Autodesk Fusion 360 part; units mm, degrees
sketch "Sketch1" plane through (0, 0, 0) normal (0, 0, 1) x (1, 0, 0)
  line L0 (0, 0) -> (169.51, 0)
  line L1 (169.51, 0) -> (169.51, 124.6)
  line L2 (169.51, 124.6) -> (0, 124.6)
  line L3 (0, 124.6) -> (0, 0)
  dimension "d1" = 169.51
  dimension "d2" = 124.6
extrude "Extrude1" add sketch "Sketch1" along normal blind 9.2 makes body 1
sketch "Sketch2" plane through (0, 0, 9.2) normal (0, 0, 1) x (-1, 0, 0)
  line L0 (0, -124.6) -> (0, 0)
  line L1 (0, 0) -> (-169.51, 0)
  line L2 (-169.51, 0) -> (-169.51, -124.6)
  line L3 (-169.51, -124.6) -> (0, -124.6)
  line L4 (-1.5, -10.3) -> (-168.01, -10.3)
  line L5 (-168.01, -10.3) -> (-168.01, -113)
  line L6 (-168.01, -113) -> (-1.5, -113)
  line L7 (-1.5, -113) -> (-1.5, -10.3)
  dimension "d5" = 1.5
  dimension "d6" = 1.5
  dimension "d7" = 11.6
  dimension "d8" = 10.3
extrude "Extrude2" cut sketch "Sketch2" against normal blind 7.6 contours L4 L5 L6 L7 bodies 1
sketch "Sketch3" plane through (0, 0, 1.6) normal (0, 0, 1) x (-1, 0, 0)
  line L0 (-1.5, -113) -> (-1.5, -10.3)
  line L1 (-1.5, -10.3) -> (-168.01, -10.3)
  line L2 (-168.01, -10.3) -> (-168.01, -113)
  line L3 (-168.01, -113) -> (-1.5, -113)
  line L4 (-8.2, -19.7) -> (-163.91, -19.7)
  line L5 (-163.91, -19.7) -> (-163.91, -105.62)
  line L6 (-163.91, -105.62) -> (-8.2, -105.62)
  line L7 (-8.2, -105.62) -> (-8.2, -19.7)
  dimension "d12" = 85.92
  dimension "d13" = 9.4
  dimension "d14" = 6.7
  dimension "d15" = 4.1
extrude "Extrude3" cut sketch "Sketch3" against normal blind 1.6 contours L4 L5 L6 L7 bodies 1
extrude "Extrude4" cut 1 faces at (59.2367, 13.4333, 1.6) along direction (0, 0, -1) blind 0.1 on bodies 1 bodies 1
sketch "Sketch4" plane through (0, 0, 1.5) normal (0, 0, 1) x (-1, 0, 0)
  line L0 (-163.91, -19.7) -> (-8.2, -19.7)
  line L1 (-8.2, -19.7) -> (-8.2, -105.62)
  line L2 (-8.2, -105.62) -> (-163.91, -105.62)
  line L3 (-163.91, -105.62) -> (-163.91, -19.7)
  line L4 (-1.5, -113) -> (-1.5, -10.3)
  line L5 (-1.5, -10.3) -> (-168.01, -10.3)
  line L6 (-168.01, -10.3) -> (-168.01, -113)
  line L7 (-168.01, -113) -> (-1.5, -113)
  line L8 (-8.2, -105.62) -> (-163.9, -105.62)
  line L9 (-163.9, -105.62) -> (-163.9, -108.4)
  line L10 (-163.9, -108.4) -> (-8.2, -108.4)
  line L11 (-8.2, -108.4) -> (-8.2, -105.62)
  dimension "d20" = 4.6
  dimension "d21" = 155.7
extrude "Extrude5" cut sketch "Sketch4" against normal blind 1.5 contours L2 L8 L9 L10 L11 bodies 1
ref_plane "WorkPlane1" through (90, 0, 0) normal (1, 0, 0) x (0, 1, 0)
split "Split1" by plane through (90, 0, 0) normal (1, 0, 0) bodies 1 makes body 2 at (141.14, 6.5667, 0)
move_body "Move1" bodies 2 to x (1, 0, 0) y (0, 1, 0) z (0, 0, 1) at (2, 0, 0)
extrude "Extrude6" add 2 faces at (90, 3.4333, 3.5667) (90, 120.7333, 3.5667) along direction (1, 0, 0) blind 2 on bodies 1 bodies 1 2
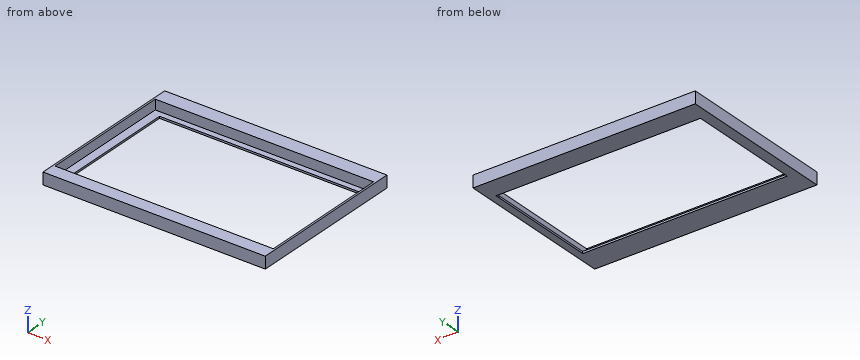
Geometry check sheet. Reference: the model listing, model coordinates, mm. Give positions to 0.01 mm unless a question says otherwise; leave off trailing zeros. Write each loop counter-clockwise with the first axis right and the second up, starting at its lowest first coordinate (ties: lowest second). Pieces come first, ordered by that corner, then holes.
1) Section check D-D, the plane y = 111. Record the boundary of the cut face in (x, z), and give its area (3 significant figures).
2) Gauge pin test, flat end, axial feed: pin 1 (3 mm diameter, centred on x = 46.5, y = 14, fed in from +Z). Record the tip position at first contact, or that the pin passes through.
3) Section check B-B, the plane z = 7.5. Record the boundary of the cut face in (x, y).
4) Section check A-A, the plane y = 56. Record the boundary of the cut face in (x, z), and give its area (3 significant figures).
5) Material ranges on L1, parallel to Y at x = 114, z = 3.5; L2, parallel to X at y = 55, z = 6.75; L3, parallel to Y at x = 12, z = 1, recorded low to high.
6) Section check C-C, the plane x = 146.5. Record the boundary of the cut face in (y, z).
Computed:
1. outline: (0, 0) - (171.51, 0) - (171.51, 9.2) - (170.01, 9.2) - (170.01, 1.5) - (1.5, 1.5) - (1.5, 9.2) - (0, 9.2) - close
1. area: 280 mm2
2. pin 1: stops at z = 1.5
3. outline: (0, 0) - (171.51, 0) - (171.51, 124.6) - (0, 124.6) - close; hole (1.5, 10.3) - (170.01, 10.3) - (170.01, 113) - (1.5, 113) - close
4. outline: (0, 0) - (8.2, 0) - (8.2, 1.5) - (1.5, 1.5) - (1.5, 9.2) - (0, 9.2) - close; (165.91, 0) - (171.51, 0) - (171.51, 9.2) - (170.01, 9.2) - (170.01, 1.5) - (165.91, 1.5) - close
4. area: 43.8 mm2
5. L1: y = 0 to 10.3, 113 to 124.6
5. L2: x = 0 to 1.5, 170.01 to 171.51
5. L3: y = 0 to 19.7, 108.4 to 124.6
6. outline: (0, 0) - (19.7, 0) - (19.7, 1.5) - (10.3, 1.5) - (10.3, 9.2) - (0, 9.2) - close; (108.4, 0) - (124.6, 0) - (124.6, 9.2) - (113, 9.2) - (113, 1.5) - (108.4, 1.5) - close
